from build123d import *

# Parameters (mm, degrees)
ESQUISSE1_W               = 8
ESQUISSE1_H               = 3
T_LE_DE_BASE_PLI_E1_DEPTH = 3


# Sheet-metal steps are written as plain solids
with BuildPart() as part:
    # Esquisse1 → Tôle de base pliée1 (new body)
    with BuildSketch(Plane.XY):
        with BuildLine():
            Line((1127.943508916, 1917.30650062), (1152.943508916, 1917.30650062))
            Line((1152.943508916, 1917.30650062), (1152.943508916, 1914.00650062))
            Line((1152.943508916, 1914.00650062), (1155.54275991, 1914.00650062))
            ThreePointArc((1155.54275991, 1914.00650062), (1155.896313301, 1913.860054011), (1156.04275991, 1913.50650062))
            Line((1156.04275991, 1913.50650062), (1156.04275991, 1912.309090129))
            ThreePointArc((1156.04275991, 1912.309090129), (1156.236433485, 1911.717619339), (1156.742435301, 1911.355253073))
            ThreePointArc((1156.742435301, 1911.355253073), (1157.511445693, 1910.806601852), (1157.810195296, 1909.910418936))
            ThreePointArc((1157.810195296, 1909.910418936), (1157.306705477, 1908.592046054), (1156.043508916, 1907.962805635))
            Line((1156.043508916, 1907.962805635), (1156.043508916, 1909.371416958))
            Line((1156.043508916, 1909.371416958), (1152.943508916, 1909.371416958))
            Line((1152.943508916, 1909.371416958), (1152.943508916, 1907.962805635))
            Line((1152.943508916, 1907.962805635), (1127.943508916, 1907.962805635))
            Line((1127.943508916, 1907.962805635), (1127.943508916, 1909.371416958))
            Line((1127.943508916, 1909.371416958), (1124.843508916, 1909.371416958))
            Line((1124.843508916, 1909.371416958), (1124.843508916, 1907.962805635))
            ThreePointArc((1124.843508916, 1907.962805635), (1123.580312356, 1908.592046054), (1123.076822537, 1909.910418936))
            ThreePointArc((1123.076822537, 1909.910418936), (1123.37557214, 1910.806601852), (1124.144582531, 1911.355253073))
            ThreePointArc((1124.144582531, 1911.355253073), (1124.650584348, 1911.717619339), (1124.844257922, 1912.309090129))
            Line((1124.844257922, 1912.309090129), (1124.844257922, 1913.50650062))
            ThreePointArc((1124.844257922, 1913.50650062), (1124.990704532, 1913.860054011), (1125.344257922, 1914.00650062))
            Line((1125.344257922, 1914.00650062), (1127.943508916, 1914.00650062))
            Line((1127.943508916, 1914.00650062), (1127.943508916, 1917.30650062))
        make_face()
        with Locations((1140.443508916, 1912.662805635)):
            Rectangle(ESQUISSE1_W, ESQUISSE1_H, mode=Mode.SUBTRACT)
    extrude(amount=-T_LE_DE_BASE_PLI_E1_DEPTH)


solid = part.part
Could you check a few things on this model? Use its own coordinates, in mm. A direction names the side the tool comes from. Coordinates: 2 decimals unless noted, no trailing zeros. Order: outer loops, then holes, each group sorted by start corner. A loop starts at its lowest first (then second) coordinate and runs counter-clockwise, first axis right, second up.
Q1. Suppose I cut it at C-C on y = 1909. Please give me the cut outline in (x, z), and give its area (3 significant figures).
Q2. Suppose I cut it at B-B on z = -2.6. Please give me the cut outline in (x, y), and give its area (3 significant figures).
Q3. Suppose I cut it at D-D on y = 1912. Please give me the cut outline in (x, z).
Q4. Which directions (+Z, -Z, +X, -X, +Y, -Y) give clear straight access to the entire face, cutting with the end or side of a thin tool? Please do faces 1 (the flat face through (1126, 1909.371, -1)), 2 (the flat face through (1136.444, 1913, -1)), 3 (the flat face through (1127.944, 1916, -1)).
Q5. Suppose I cut it at A-A on x = 1137. Please give me the cut outline in (y, z), and give its area (3 significant figures).
Q6. Thinking about a two-plate mould opening in X: for faces 4 (the cylindrical face through (1157.5, 1910.82, -1.48)), 5 (the cylindrical face through (1123.59, 1908.58, -1.48)), 6 (the flat face through (1127.944, 1909, -1)), which applies, released by +X, released by -X, zero draft, split by the parting line, or undercut?
Q7. Will these pins go through, and if not, where does the flat tip stop? pin 1 (1 mm diameter, centred on y = 1916, z = -1, fed in from -X); pin 2 (1.5 mm diameter, centred on x = 1126.5, z = -1.5, fed in from -Y); pin 3 (0.7 mm diameter, centred on y = 1909, z = -2, fed in from +X).
Q8. Please list where these lines run through material, in increasing order: L1, parallel to X at y = 1908.75, z = -0.9; L2, parallel to Y at x = 1144, z = -0.2; L3, parallel to X at y = 1912.5, z = -0.25.
Answer:
1. outline: (1123.3, -3) - (1124.84, -3) - (1124.84, 0) - (1123.3, 0) - close; (1127.94, -3) - (1152.94, -3) - (1152.94, 0) - (1127.94, 0) - close; (1156.04, -3) - (1157.59, -3) - (1157.59, 0) - (1156.04, 0) - close
1. area: 84.3 mm2
2. outline: (1123.08, 1909.91) arc R1.94 ccw to (1124.84, 1907.96) - (1124.84, 1909.37) - (1127.94, 1909.37) - (1127.94, 1907.96) - (1152.94, 1907.96) - (1152.94, 1909.37) - (1156.04, 1909.37) - (1156.04, 1907.96) arc R1.94 ccw to (1157.81, 1909.91) arc R1.53 ccw to (1156.74, 1911.36) arc R1 cw to (1156.04, 1912.31) - (1156.04, 1913.51) arc R0.5 ccw to (1155.54, 1914.01) - (1152.94, 1914.01) - (1152.94, 1917.31) - (1127.94, 1917.31) - (1127.94, 1914.01) - (1125.34, 1914.01) arc R0.5 ccw to (1124.84, 1913.51) - (1124.84, 1912.31) arc R1 cw to (1124.14, 1911.36) arc R1.53 ccw to start; hole (1136.44, 1911.16) - (1144.44, 1911.16) - (1144.44, 1914.16) - (1136.44, 1914.16) - close
2. area: 248 mm2
3. outline: (1124.8, -3) - (1136.44, -3) - (1136.44, 0) - (1124.8, 0) - close; (1144.44, -3) - (1156.09, -3) - (1156.09, 0) - (1144.44, 0) - close
4. face 1: +Z, -Z, -Y
4. face 2: +Z, -Z
4. face 3: +Z, -Z, -X, +Y
5. outline: (1907.96, -3) - (1911.16, -3) - (1911.16, 0) - (1907.96, 0) - close; (1914.16, -3) - (1917.31, -3) - (1917.31, 0) - (1914.16, 0) - close
5. area: 19.0 mm2
6. face 4: released by +X
6. face 5: released by -X
6. face 6: undercut
7. pin 1: stops at x = 1127.94
7. pin 2: stops at y = 1909.37
7. pin 3: stops at x = 1157.73
8. L1: x = 1123.45 to 1124.84, 1127.94 to 1152.94, 1156.04 to 1157.44
8. L2: y = 1907.96 to 1911.16, 1914.16 to 1917.31
8. L3: x = 1124.84 to 1136.44, 1144.44 to 1156.04
